Source: CAD feature listing. Evaluate the final solid. Frame: model axes, mm. Face numbers are marked on the shaded views. Give positions to 0.01 mm unless a question says otherwise; leave off trailing zeros. Write each loop counter-clockwise with the first axis right and the second up, starting at its lowest first coordinate (ties: lowest second). Pieces come first, ordered by that corner, then holes. Notation, with made-up numbers: M -37,55 L -19,55 A27 cw -19,71 Z; hole C 39,34 d9. An arc over 180 degrees is marked long. Return JSON: item names as keys, results as strings.
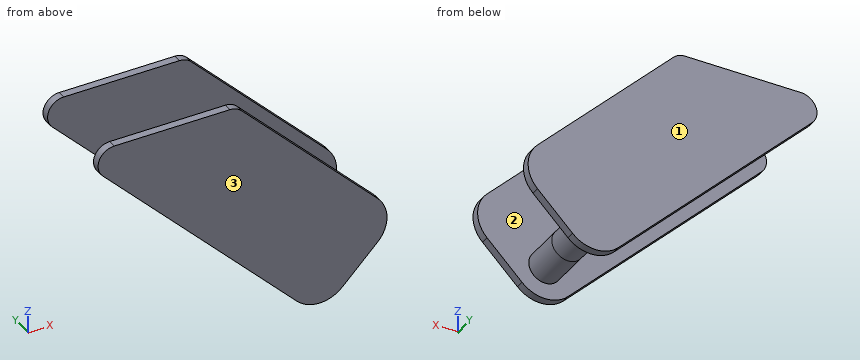
```python
from build123d import *

# Parameters (mm, degrees)
F2_DEPTH = 5
F3_R     = 10
F4_DEPTH = 25


with BuildPart() as f2:
    # F1 (on offset) → F2 (new body)
    with BuildSketch(Plane.XZ.offset(25)):
        with BuildLine():
            Line((-4.142136, 50), (-75.857864, 50))
            ThreePointArc((-75.857864, 50), (-85.09666, 43.826834), (-82.928932, 32.928932))
            Line((-82.928932, 32.928932), (37.279221, -87.279221))
            ThreePointArc((37.279221, -87.279221), (51.421356, -93.137085), (65.563492, -87.279221))
            Line((65.563492, -87.279221), (87.279221, -65.563492))
            ThreePointArc((87.279221, -65.563492), (93.137085, -51.421356), (87.279221, -37.279221))
            Line((87.279221, -37.279221), (2.928932, 47.071068))
            ThreePointArc((2.928932, 47.071068), (-0.315301, 49.238795), (-4.142136, 50))
        make_face()
    extrude(amount=F2_DEPTH)

    # F3 (on face) → F4 (join)
    with BuildSketch(Plane(origin=(0, -25, 0), x_dir=(-1, 0, 0), z_dir=(0, 1, 0))):
        with Locations((-51.421356, -73.137085)):
            Circle(F3_R)
    extrude(amount=F4_DEPTH)

    # F5: F2 across plane


with BuildPart() as f2_1:
    add(f2.part)
    add(f2.part.mirror(Plane.XZ))


solid = f2_1.part
```
1) Contact query for flat-ended pins moving along their axis: pin 1 Ø10 at (x, y) = (56, -7.5) entering from +Z; pin 2 Ø6 at (y, z) = (24, -51) entering from +X; pin 3 Ø10 at (y, z) = (23.5, 3) entering from -X. Output: stop coordinate, or through.
Numbers:
{"pin 1": "stops at z = -63.14", "pin 2": "stops at x = 93.14", "pin 3": "stops at x = -57.77"}
2) Line query: line 1 (Y direction, x = -27, z = 33.5); line 2 (X direction, y = 23, z = -75.5); line 3 (Z direction, x = 6, y = -26). Output: solid intervals per line, ascending. Write a range as [from, to].
Numbers:
{"line 1": "y = [-30, -25], [25, 30]", "line 2": "x = [41.7, 61.14]", "line 3": "z = [-56, 44]"}
3) Cut plane C-C, the plane z = -68.5. Return the cut outline in (x, y), then the cut area to 3 significant figures.
Numbers:
{"outline": "M 18.5,-30 L 84.34,-30 L 84.34,-25 L 60.28,-25 L 60.28,25 L 84.34,25 L 84.34,30 L 18.5,30 L 18.5,25 L 42.56,25 L 42.56,-25 L 18.5,-25 Z", "area": "1,540 mm²"}
4) Cut plane A-A, the plane x = -38.5. Return the cut outline in (y, z).
Numbers:
{"outline": "M -30,-11.5 L -25,-11.5 L -25,50 L -30,50 Z; M 25,-11.5 L 30,-11.5 L 30,50 L 25,50 Z"}
5) Draft query along Y for the marked faces 1, 2 and 3. Return one class per face: released by +Y, released by -Y, zero draft, split by the parting line, or undercut.
Numbers:
{"face 1": "released by +Y", "face 2": "undercut", "face 3": "released by -Y"}
6) Cut plane D-D, the plane x = 47. Return the cut outline in (y, z).
Numbers:
{"outline": "M -30,-92.64 L -25,-92.64 L -25,-82.11 L 25,-82.11 L 25,-92.64 L 30,-92.64 L 30,3 L 25,3 L 25,-64.17 L -25,-64.17 L -25,3 L -30,3 Z"}
7) Cut plane B-B, the plane z = -14.5. Return the cut outline in (x, y).
Numbers:
{"outline": "M -35.5,-30 L 64.5,-30 L 64.5,-25 L -35.5,-25 Z; M -35.5,25 L 64.5,25 L 64.5,30 L -35.5,30 Z"}
